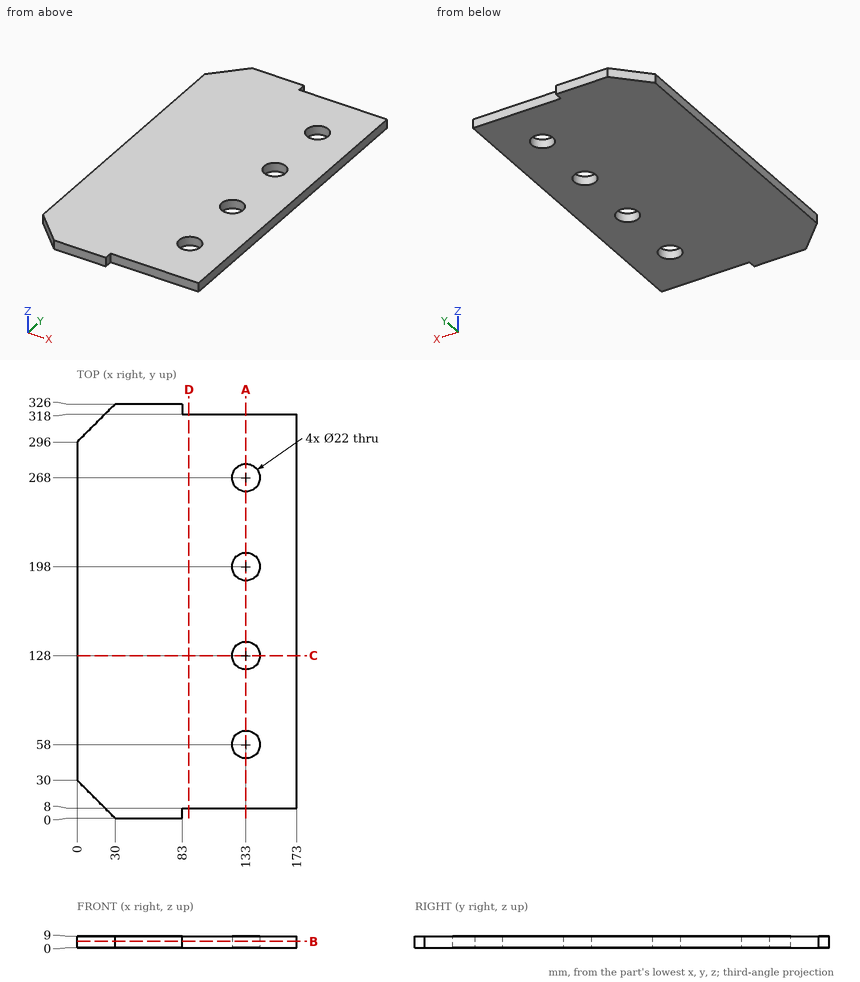
Could you check a few things on this drawing? It's one solid part, dimensions in mm from its lowest x, y, z. Give positions to 0.01 mm unless a question says otherwise; leave off trailing zeros. Loops run counter-clockwise (first coordinate to the right, second up) from the corner with the lowest first, then second, coordinate; pieces in that order, holes last. Notation, with made-up numbers: M 76.5,18 L 80.5,18 A11 cw 80.5,22 Z; hole C 3,-18.75 d2. An arc over 180 degrees is marked long. Answer as a JSON object with one key per item and string values.
Q1. Suppose I cut it at A-A, the plane x = 133. List the corners of the cut face in (y, z) for me.
Values found:
{"outline": "M 8,0 L 47,0 L 47,9 L 8,9 Z; M 69,0 L 117,0 L 117,9 L 69,9 Z; M 139,0 L 187,0 L 187,9 L 139,9 Z; M 209,0 L 257,0 L 257,9 L 209,9 Z; M 279,0 L 318,0 L 318,9 L 279,9 Z"}
Q2. Suppose I cut it at D-D, the plane x = 88. List the corners of the cut face in (y, z) for me.
Values found:
{"outline": "M 8,0 L 318,0 L 318,9 L 8,9 Z"}
Q3. If I drill on probe 1 along Y at (x, z) = (133, 3); probe 2 along X at (y, z) = (128, 5.75); probe 3 along Y at (x, z) = (123.5, 5.75), over which ranges is the centre line in solid material (lowest first)? Write a range as [from, to].
Values found:
{"probe 1": "y = [8, 47], [69, 117], [139, 187], [209, 257], [279, 318]", "probe 2": "x = [0, 122], [144, 173]", "probe 3": "y = [8, 52.45], [63.55, 122.45], [133.55, 192.45], [203.55, 262.45], [273.55, 318]"}
Q4. For P1, Ø4.5, axis at x = 117, z = 4, coming from the -Y side, with a flat end and sliding along its axis, tell me the tip position at first contact or that it passes through.
Values found:
{"P1": "stops at y = 8"}
Q5. Suppose I cut it at C-C, the plane y = 128. List the corners of the cut face in (x, z) for me, plus the area to 3 significant figures.
Values found:
{"outline": "M 0,0 L 122,0 L 122,9 L 0,9 Z; M 144,0 L 173,0 L 173,9 L 144,9 Z", "area": "1,360 mm²"}
Q6. Suppose I cut it at B-B, the plane z = 5. List the corners of the cut face in (x, y) for me, plus the area to 3 significant figures.
Values found:
{"outline": "M 0,30 L 30,0 L 83,0 L 83,8 L 173,8 L 173,318 L 83,318 L 83,326 L 30,326 L 0,296 Z; hole C 133,58 d22; hole C 133,128 d22; hole C 133,198 d22; hole C 133,268 d22", "area": "52,500 mm²"}
